from build123d import *

# Parameters (mm, degrees)
SKETCH1_R           = 15
SKETCH1_R_2         = 11.25
BOSS_EXTRUDE1_DEPTH = 8
SKETCH1_3_R         = 11.25
SKETCH1_3_R_2       = 6.35
BOSS_EXTRUDE2_DEPTH = 2
FILLET1_R           = 1


with BuildPart() as part:
    # Sketch1 → Boss-Extrude1 (new body)
    with BuildSketch(Plane.XY):
        Circle(SKETCH1_R)
        Circle(SKETCH1_R_2, mode=Mode.SUBTRACT)
    extrude(amount=BOSS_EXTRUDE1_DEPTH)

    # Sketch1<3> → Boss-Extrude2 (add)
    with BuildSketch(Plane.XY):
        Circle(SKETCH1_3_R)
        Circle(SKETCH1_3_R_2, mode=Mode.SUBTRACT)
    extrude(amount=BOSS_EXTRUDE2_DEPTH)

    # Fillet1
    fillet1_edges = [part.edges().sort_by_distance(p)[0] for p in [
        (-15, 0, 8),
        (-15, 0, 0),
        (-11.25, 0, 8),
    ]]
    fillet(fillet1_edges, radius=FILLET1_R)


solid = part.part
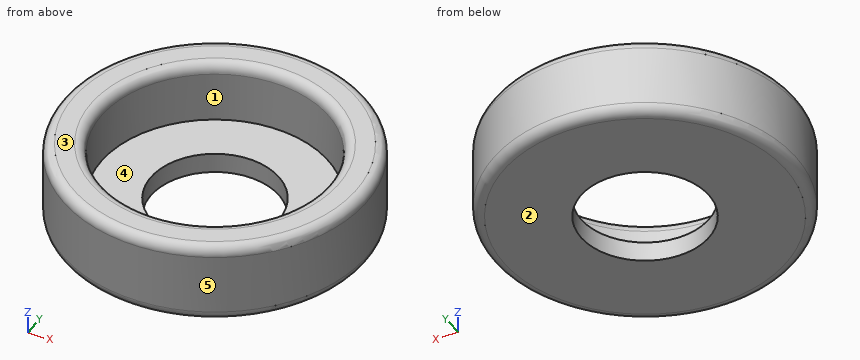
Model file for the job. Use its own axes, mm. Face numbers are marked on the shaded views. A direction names the side the tool comes from. Round coordinates to 2 decimals unless told otherwise and drop trailing zeros. Loops run counter-clockwise (first coordinate to the right, second up) from the corner with the lowest first, then second, coordinate; pieces in that order, holes last. Notation, with made-up numbers: (80.25, -21.5) - (139.25, -21.5) arc R32 cw to (139.25, 15.5) - close; hole circle Ø7 at (-29, 16.25). An arc over 180 degrees is marked (long way). Write each question's results on one line, items separated by ' | '.
(1) Wall check: L1, parallel to Y at x = 0, z = 5.05; L2, parallel to Y at x = -5.25, z = 5; L3, parallel to Z at x = 12.25, y = -7. Give the ranges that are in metal, low to high.
Answer below:
L1: y = -15 to -11.25, 11.25 to 15 | L2: y = -14.05 to -9.95, 9.95 to 14.05 | L3: z = 0.01 to 7.99
(2) Saw through at B-B, the plane z = 6.5. List the corners of the cut face in (x, y).
Answer below:
outline: circle Ø30 at (0, 0); hole circle Ø22.5 at (0, 0)
(3) Mould opens along Y. For the marked faces 3, 4 and 5 say: released by +Y, released by -Y, zero draft, split by the parting line, or undercut.
Answer below:
face 3: zero draft | face 4: undercut | face 5: split by the parting line
(4) Pin check, flat tips, straight feed: pin 1 (3 mm diameter, centred on x = -11.5, z = 6.5, fed in from -Y); pin 2 (3 mm diameter, centred on y = 6.5, z = 4.5, fed in from +X); pin 3 (4 mm diameter, centred on x = -11.5, y = -11, fed in from -Z); pin 4 (3 mm diameter, centred on x = 10.5, z = 2, fed in from +Y). Stop position of each tip, or through.
Answer below:
pin 1: stops at y = -11.18 | pin 2: stops at x = 14.14 | pin 3: stops at z = 0 | pin 4: stops at y = 12
(5) Saw through at A-A, the plane x = 0. List the corners of the cut face in (y, z), then the cut area to 3 significant figures.
Answer below:
outline: (-15, 1) arc R1 ccw to (-14, 0) - (-6.35, 0) - (-6.35, 2) - (-11.25, 2) - (-11.25, 7) arc R1 ccw to (-12.25, 8) - (-14, 8) arc R1 ccw to (-15, 7) - close; (6.35, 0) - (14, 0) arc R1 ccw to (15, 1) - (15, 7) arc R1 ccw to (14, 8) - (12.25, 8) arc R1 ccw to (11.25, 7) - (11.25, 2) - (6.35, 2) - close | area: 78.3 mm^2
(6) 3-axis set-ups, long thin cutter, end or side, ignore diameter. For the marked faces 1 and 2: which of +Z, -Z, +X, -X, +Y, -Y reach the whole face in a straight line?
Answer below:
face 1: +Z | face 2: -Z, +X, -X, +Y, -Y
(7) Saw through at C-C, the plane z = 1.5. List the corners of the cut face in (x, y), then the cut area to 3 significant figures.
Answer below:
outline: circle Ø30 at (0, 0); hole circle Ø12.7 at (0, 0) | area: 580 mm^2
